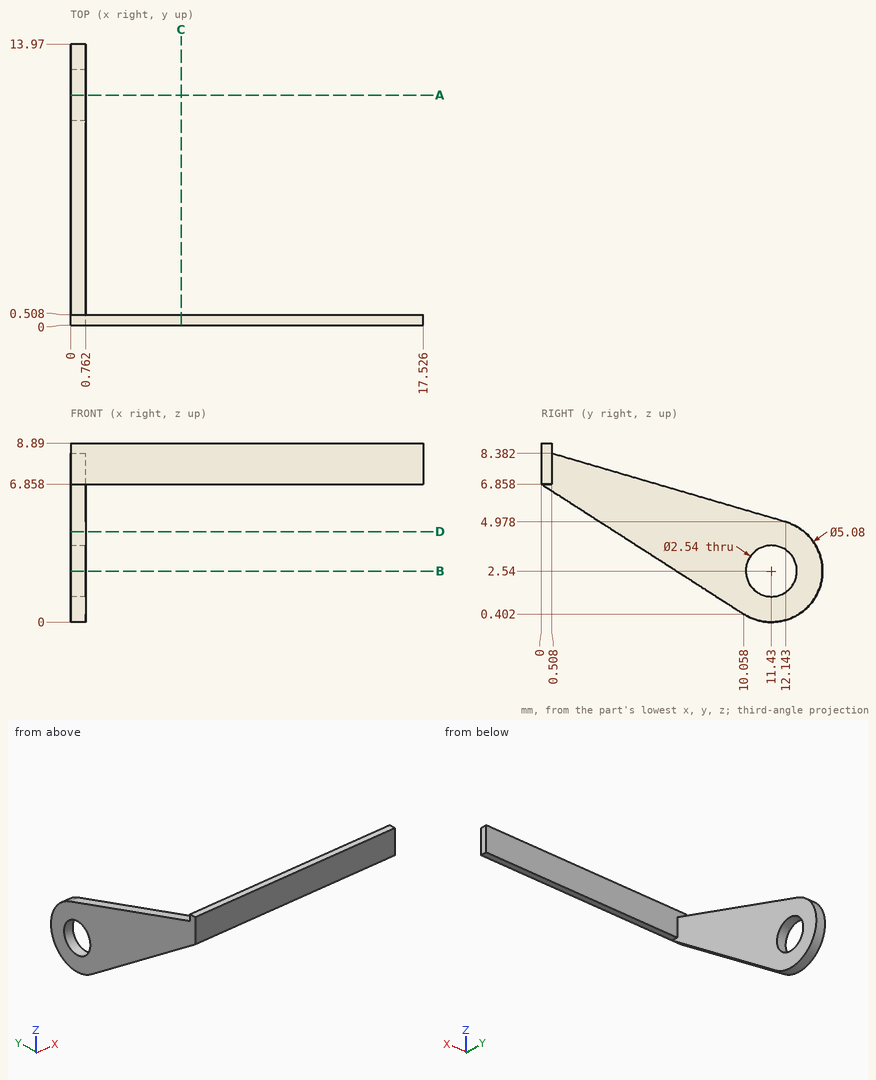
Geometry: see drawing. Coordinates: mm, zero at the bounding-box minimum. Round coordinates to 2 decimals unless told otherwise and drop trailing zeros. Write each loop counter-clockwise with the first axis right and the second up, starting at its lowest first coordinate (ties: lowest second). Pieces come first, ordered by that corner, then holes.
Item 1: Section query A-A (y = 11.43). Return loops of the section in (x, z).
Item 2: Material intervals for L1, parallel to Y at x = 2, z = 8.25; L2, parallel to X at y = 12.25, z = 4; L3, parallel to Y at x = 0.5, z = 2.54 (1 decimal), sorted ascending.
Item 3: Section query B-B (z = 2.54). Return loops of the section in (x, y).
Item 4: Section query C-C (x = 5.5). Return loops of the section in (y, z).
Item 5: Pin query (flat end, axial travel): P1, Ø2, axis at y = 11.43, z = 2.54, coming from the +X side (3 decimals); P2, Ø0.6, axis at x = 10.5, y = 0.5, coming from the -Z side; P3, Ø2.5, axis at y = 4, z = 3, coming from the +X side; P4, Ø2, axis at x = 12.5, z = 8.5, coming from the +Y side. Return the tip coordinate at first contact, or that it passes through.
Item 6: Section query D-D (z = 4.5). Return loops of the section in (x, y) (1 decimal).
Completed:
1. outline: (0, 0) - (0.76, 0) - (0.76, 1.27) - (0, 1.27) - close; (0, 3.81) - (0.76, 3.81) - (0.76, 5.19) - (0, 5.19) - close
2. L1: y = 0 to 0.51
2. L2: x = 0 to 0.76
2. L3: y = 6.7 to 10.2, 12.7 to 14
3. outline: (0, 6.73) - (0.76, 6.73) - (0.76, 10.16) - (0, 10.16) - close; (0, 12.7) - (0.76, 12.7) - (0.76, 13.97) - (0, 13.97) - close
4. outline: (0, 6.86) - (0.51, 6.86) - (0.51, 8.89) - (0, 8.89) - close
5. P1: passes through
5. P2: stops at z = 6.86
5. P3: stops at x = 0.76
5. P4: stops at y = 0.51
6. outline: (0, 3.7) - (0.8, 3.7) - (0.8, 13) - (0, 13) - close
